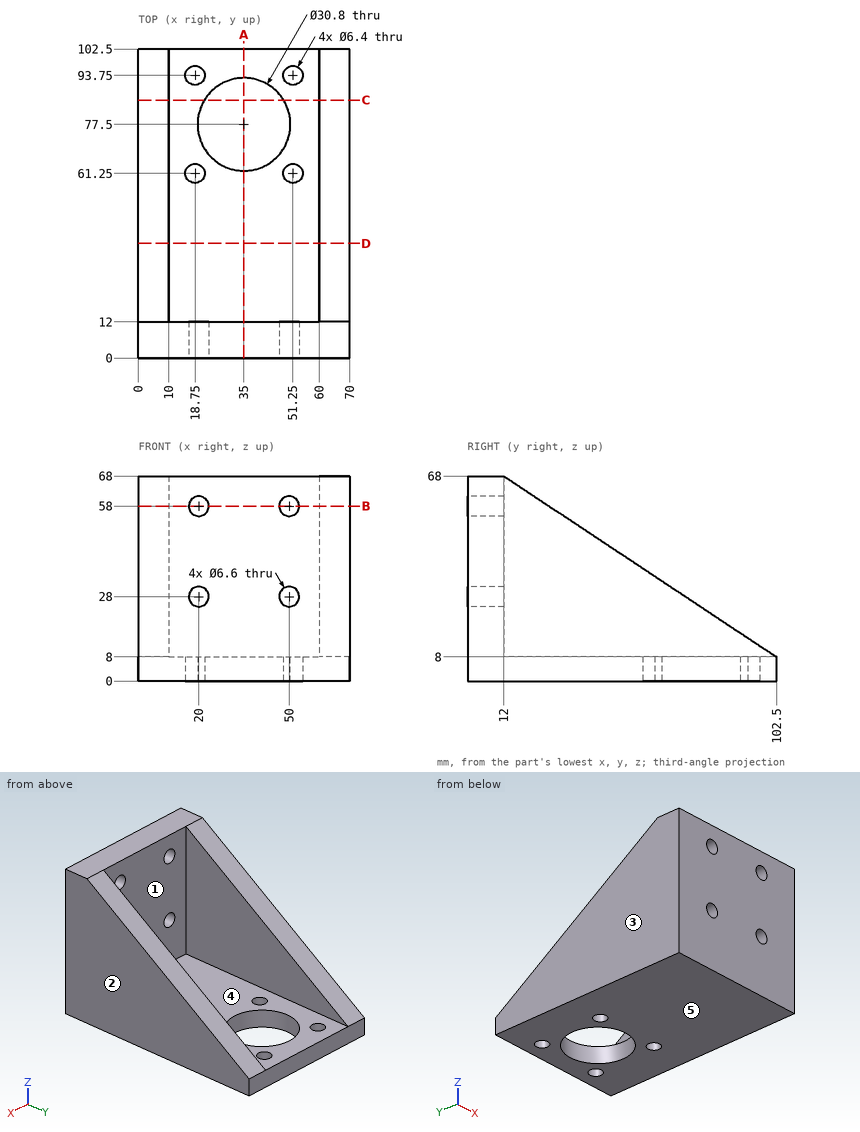
Input: dimensioned drawing with shaded views. Units: mm. Origin: part minimum x, y, z. A direction names the side the tool comes from. Coordinates: 2 decimals unless noted, no trailing zeros. Order: outer loops, then holes, each group sorted by start corner. A loop starts at its lowest first (then second) coordinate and runs counter-clockwise, first axis right, second up.
Item 1: Section query A-A (x = 35). Output: boundary loops of the cut face in (y, z), then the cut area to 3 significant figures.
Answer:
outline: (0, 0) - (62.1, 0) - (62.1, 8) - (12, 8) - (12, 68) - (0, 68) - close; (92.9, 0) - (102.5, 0) - (102.5, 8) - (92.9, 8) - close
area: 1,290 mm2
Item 2: Access query for the marked faces 4 and 5. Directions: +Z, -Z, +X, -X, +Y, -Y. A direction counts if a zero-diameter tool reaches every point of the face in a straight line with its end or side. Return the directions, or none.
Answer:
face 4: +Z, +Y
face 5: -Z, +X, -X, +Y, -Y
Item 3: Section query C-C (y = 85.5). Output: boundary loops of the cut face in (x, z), then the cut area to 3 significant figures.
Answer:
outline: (0, 0) - (21.84, 0) - (21.84, 8) - (10, 8) - (10, 19.27) - (0, 19.27) - close; (48.16, 0) - (70, 0) - (70, 19.27) - (60, 19.27) - (60, 8) - (48.16, 8) - close
area: 575 mm2
Item 4: Section query B-B (z = 58). Output: boundary loops of the cut face in (x, y), then the cut area to 3 significant figures.
Answer:
outline: (0, 0) - (16.7, 0) - (16.7, 12) - (10, 12) - (10, 27.08) - (0, 27.08) - close; (23.3, 0) - (46.7, 0) - (46.7, 12) - (23.3, 12) - close; (53.3, 0) - (70, 0) - (70, 27.08) - (60, 27.08) - (60, 12) - (53.3, 12) - close
area: 983 mm2
Item 5: Draft query along X for the marked faces 1, 2 and 3. Return one class per face: released by +X, released by -X, zero draft, split by the parting line, or undercut.
Answer:
face 1: undercut
face 2: released by +X
face 3: released by -X
Item 6: Material intervals for line 1 along X through (y, z) = (61.25, 2.75); line 2 along X through (y, z) = (29, 27); line 3 along Z through (x, y) = (50, 8.25), sorted ascending.
Answer:
line 1: x = 0 to 15.55, 21.95 to 48.05, 54.45 to 70
line 2: x = 0 to 10, 60 to 70
line 3: z = 0 to 24.7, 31.3 to 54.7, 61.3 to 68
Item 7: Contact query for flat-ended pins moving along their axis: P1, Ø1.5, axis at x = 61.5, y = 78.5, coming from the +Z side; P2, Ø6, axis at x = 20, z = 28, coming from the +Y side; P3, Ø7.5, axis at x = 50, z = 28, coming from the +Y side; P4, Ø12, axis at x = 48, y = 54.5, coming from the +Z side. Output: stop coordinate, or through.
Answer:
P1: stops at z = 24.41
P2: passes through
P3: stops at y = 12
P4: stops at z = 8
Item 8: Section query D-D (y = 38). Output: boundary loops of the cut face in (x, z), then the cut area to 3 significant figures.
Answer:
outline: (0, 0) - (70, 0) - (70, 50.76) - (60, 50.76) - (60, 8) - (10, 8) - (10, 50.76) - (0, 50.76) - close
area: 1,420 mm2
